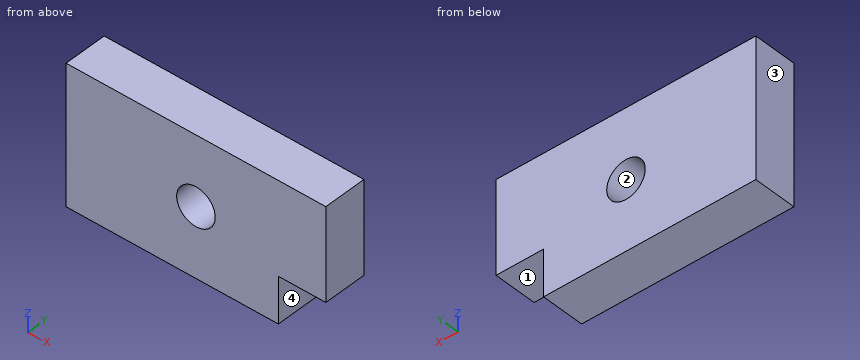
from build123d import *

# Parameters (mm, degrees)
F1_DEPTH = 50
F2_R     = 22.248347
F3_DEPTH = 50.001


with BuildPart() as f1:
    # F0 (on Front) → F1 (new body)
    with BuildSketch(Plane.XZ):
        Polygon((-150, -80), (95.169887, -80), (95.169887, -26.802706), (150, -26.802706), (150, 80), (-150, 80), align=None)
    extrude(amount=F1_DEPTH)

    # F2 (on Front) → F3 (cut, through all)
    with BuildSketch(Plane.XZ):
        Circle(F2_R)
    extrude(amount=F3_DEPTH, mode=Mode.SUBTRACT)


solid = f1.part
Here's how the part is built. I have some questions about the finished solid (model axes, mm). Face numbers are marked on the shaded views. Round coordinates to 2 decimals unless told otherwise and drop trailing zeros. Loops run counter-clockwise (first coordinate to the right, second up) from the corner with the lowest first, then second, coordinate; pieces in that order, holes last. Notation, with made-up numbers: (53, -36) -> (64, -36) arc R13 ccw to (64, -18) -> close; hole circle Ø3 at (-29.5, 38.5). An arc over 180 degrees is marked (long way). Write each question's results on one line, items separated by ' | '.
(1) If I drill on L1, parallel to X at y = -13, z = 0; L2, parallel to Z at x = 1.5, y = -18.5; L3, parallel to X at y = -13, z = -40, over which ranges is the centre line in solid material (lowest first)?
Worked answers:
L1: -150 to -22.25, 22.25 to 150 | L2: -80 to -22.2, 22.2 to 80 | L3: -150 to 95.17
(2) If we section it at A-A, the plane x = 0: List the corners of the cut face in (y, z) for me.
Worked answers:
outline: (-50, -80) -> (0, -80) -> (0, -22.25) -> (-50, -22.25) -> close; (-50, 22.25) -> (0, 22.25) -> (0, 80) -> (-50, 80) -> close
(3) We'd pull the mould along X, two halves only. Please class the marked faces 1, 2, 3 and 4: released by +X, released by -X, zero draft, split by the parting line, or undercut.
Worked answers:
face 1: zero draft | face 2: undercut | face 3: released by -X | face 4: released by +X
(4) If we section it at C-C, the plane y = -42: List the corners of the cut face in (x, z) for me.
Worked answers:
outline: (-150, -80) -> (95.17, -80) -> (95.17, -26.8) -> (150, -26.8) -> (150, 80) -> (-150, 80) -> close; hole circle Ø44.5 at (0, 0)
(5) If we section it at B-B, the plane z = 0: List the corners of the cut face in (x, y) for me, then the cut area to 3 significant figures.
Worked answers:
outline: (-150, -50) -> (-22.25, -50) -> (-22.25, 0) -> (-150, 0) -> close; (22.25, -50) -> (150, -50) -> (150, 0) -> (22.25, 0) -> close | area: 12,800 mm2
(6) For P1, Ø15, axis at x = 110.5, y = -32, coming from the -Z side, with a flat end and sliding along its axis, tell me the tip position at first contact or that it passes through.
Worked answers:
P1: z = -26.8
(7) If we section it at D-D, the plane z = -65.5: List the corners of the cut face in (x, y) for me.
Worked answers:
outline: (-150, -50) -> (95.17, -50) -> (95.17, 0) -> (-150, 0) -> close
